Answer from the drawing. Dimensions are ordinates in mm from the lowest x, y and z of the part. Coordinates: 2 decimals unless noted, no trailing zeros. Order: outer loops, then holes, each group sorted by start corner. A loop starts at its lowest first (then second) coordinate and runs counter-clockwise, first axis right, second up. Notation, with made-up numbers: (0.25, 82) -> (5.25, 82) arc R20 ccw to (5.25, 109) -> close; hole circle Ø2 at (-24.75, 9.5). An arc over 180 degrees is marked (long way). Answer in a Markdown table with one row per item.
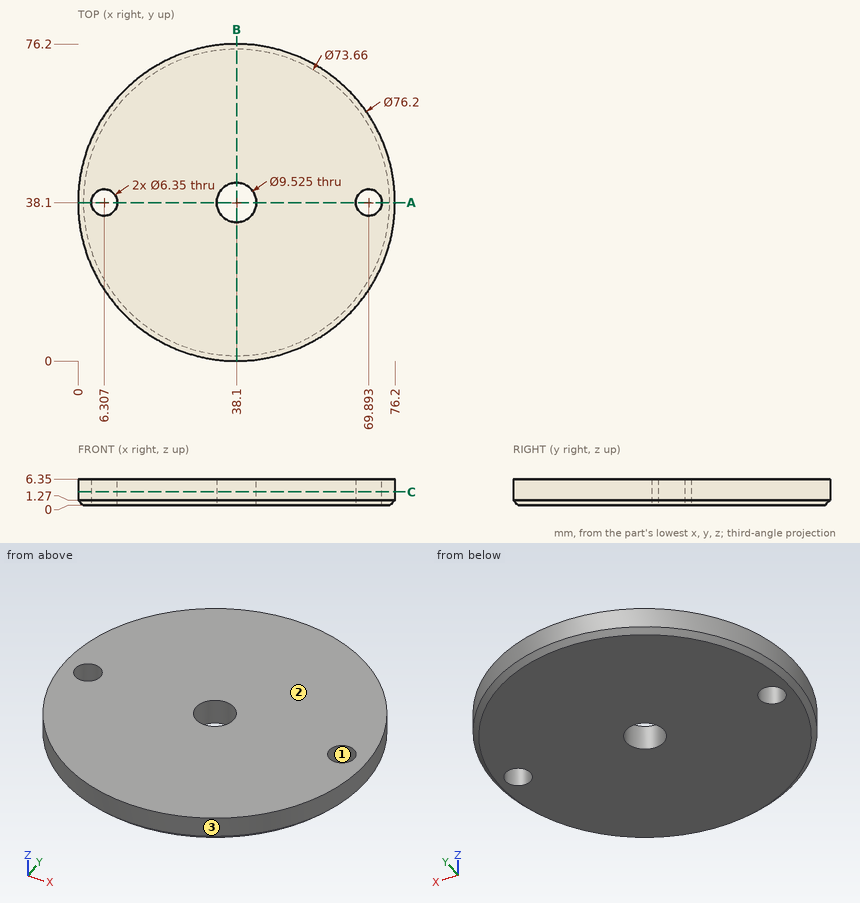
(1) A cutting plane is placed at A-A, the plane y = 38.1. Determine the outline of the cut face in (x, z), then the cut area to 3 significant figures.
Check values:
| item | result |
|---|---|
| outline | (0, 1.27) -> (1.27, 0) -> (3.13, 0) -> (3.13, 6.35) -> (0, 6.35) -> close; (9.48, 0) -> (33.34, 0) -> (33.34, 6.35) -> (9.48, 6.35) -> close; (42.86, 0) -> (66.72, 0) -> (66.72, 6.35) -> (42.86, 6.35) -> close; (73.07, 0) -> (74.93, 0) -> (76.2, 1.27) -> (76.2, 6.35) -> (73.07, 6.35) -> close |
| area | 341 mm² |
(2) A cutting plane is placed at B-B, the plane x = 38.1. Determine the outline of the cut face in (y, z), then the cut area to 3 significant figures.
Check values:
| item | result |
|---|---|
| outline | (0, 1.27) -> (1.27, 0) -> (33.34, 0) -> (33.34, 6.35) -> (0, 6.35) -> close; (42.86, 0) -> (74.93, 0) -> (76.2, 1.27) -> (76.2, 6.35) -> (42.86, 6.35) -> close |
| area | 422 mm² |
(3) Flat-ended cylindrical pins translate along their axes: pin 1 (1.5 mm diameter, centred on x = 53, z = 4.5, fed in from +Y) (1 decimal); pin 2 (5.5 mm diameter, centred on x = 6.31, y = 38.1, fed in from -Z); pin 3 (1 mm diameter, centred on x = 67.5, z = 3.5, fed in from -Y); pin 4 (3 mm diameter, centred on x = 23.5, z = 5.5, fed in from -Y). Find the tip coordinate at first contact, or state that the pin passes through.
Check values:
| item | result |
|---|---|
| pin 1 | y = 73.5 |
| pin 2 | through |
| pin 3 | y = 13.27 |
| pin 4 | y = 2.32 |
(4) Find the intervals of material crossed by line 1 along Y through (x, z) = (38.1, 4.5); line 2 along Y through (x, z) = (41, 3.75); line 3 along Y through (x, z) = (58.5, 3.5), in increasing order. Write a range as from..to.
Check values:
| item | result |
|---|---|
| line 1 | 0..33.34, 42.86..76.2 |
| line 2 | 0.11..34.32, 41.88..76.09 |
| line 3 | 5.92..70.28 |
(5) For a pull along Y with two mould halves and no side action, classify the marked faces 1, 2 and 3 as released by +Y, released by -Y, zero draft, split by the parting line, or undercut.
Check values:
| item | result |
|---|---|
| face 1 | undercut |
| face 2 | zero draft |
| face 3 | split by the parting line |
(6) A cutting plane is placed at C-C, the plane z = 3.25. Count the separate pieces of the cut face and the enclosed holes in it, then the cut area to 3 significant figures.
Check values:
| item | result |
|---|---|
| separate pieces | 1 |
| enclosed holes | 3 |
| area | 4,430 mm² |
